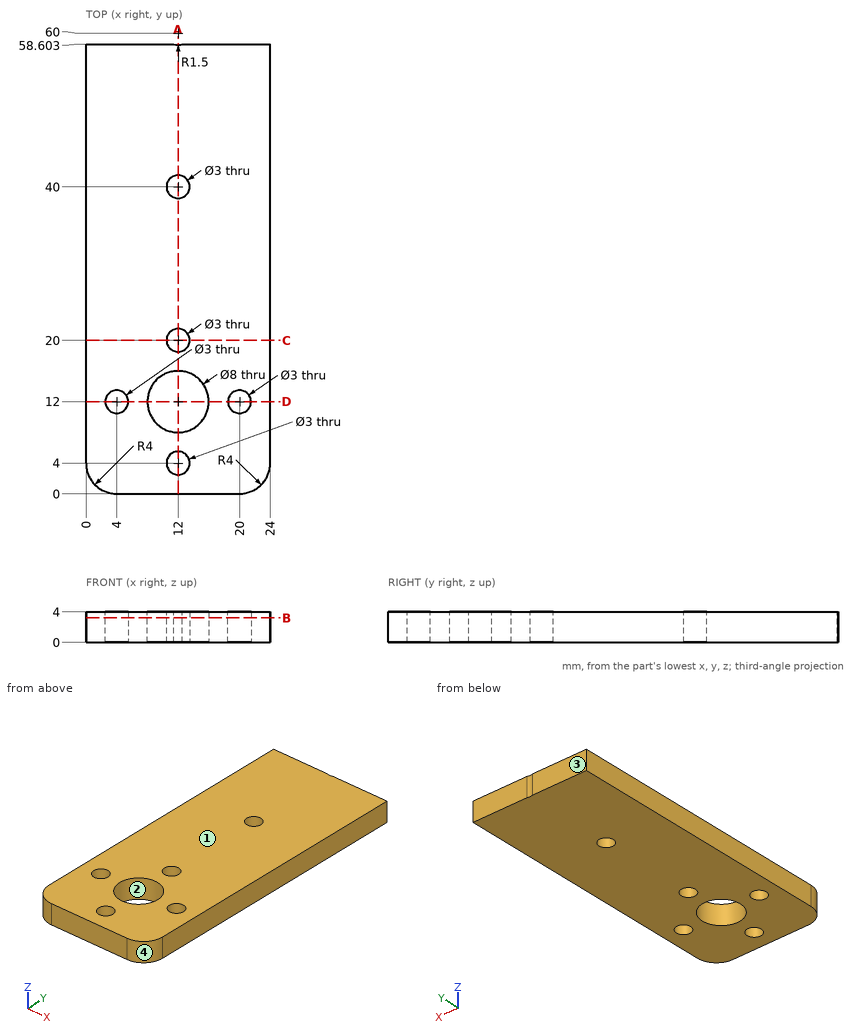
For this review, use the dimensioned drawing (mm, ordinates from the lowest corner) and the shaded views. Round coordinates to 2 decimals unless told otherwise and drop trailing zeros. Order: outer loops, then holes, each group sorted by start corner. A loop starts at its lowest first (then second) coordinate and runs counter-clockwise, first axis right, second up.
1) For L1, parallel to Y at x = 12, z = 2.4; L2, parallel to Y at x = 20, z = 1.65; L3, parallel to X at y = 11, z = 3.4, list the stretches that pass through material, from the lowest coordinate up.
The answers:
L1: y = 0 to 2.5, 5.5 to 8, 16 to 18.5, 21.5 to 38.5, 41.5 to 58.5
L2: y = 0 to 10.5, 13.5 to 58.6
L3: x = 0 to 2.88, 5.12 to 8.13, 15.87 to 18.88, 21.12 to 24
2) Clearance check with a flat-ended pin moving along its axis: pin 1 Ø5 at (x, y) = (12, 40) entering from +Z. State where the tip first meets the part, or that it passes through.
The answers:
pin 1: stops at z = 4
3) Consider section D-D (y = 12). State the section outline as (x, z) points.
The answers:
outline: (0, 0) - (2.5, 0) - (2.5, 4) - (0, 4) - close; (5.5, 0) - (8, 0) - (8, 4) - (5.5, 4) - close; (16, 0) - (18.5, 0) - (18.5, 4) - (16, 4) - close; (21.5, 0) - (24, 0) - (24, 4) - (21.5, 4) - close
4) Consider section A-A (x = 12). State the section outline as (y, z) points.
The answers:
outline: (0, 0) - (2.5, 0) - (2.5, 4) - (0, 4) - close; (5.5, 0) - (8, 0) - (8, 4) - (5.5, 4) - close; (16, 0) - (18.5, 0) - (18.5, 4) - (16, 4) - close; (21.5, 0) - (38.5, 0) - (38.5, 4) - (21.5, 4) - close; (41.5, 0) - (58.5, 0) - (58.5, 4) - (41.5, 4) - close
5) Consider section B-B (z = 3.2). State the section outline as (x, y) points, plus the area to 3 significant figures.
The answers:
outline: (0, 4) arc R4 ccw to (4, 0) - (20, 0) arc R4 ccw to (24, 4) - (24, 58.6) - (12.55, 58.6) arc R1.5 cw to (11.45, 58.6) - (0, 58.6) - close; hole circle Ø3 at (4, 12); hole circle Ø8 at (12, 12); hole circle Ø3 at (12, 4); hole circle Ø3 at (12, 20); hole circle Ø3 at (12, 40); hole circle Ø3 at (20, 12)
area: 1,310 mm2
6) Consider section C-C (y = 20). State the section outline as (x, z) points, plus the area to 3 significant figures.
The answers:
outline: (0, 0) - (10.5, 0) - (10.5, 4) - (0, 4) - close; (13.5, 0) - (24, 0) - (24, 4) - (13.5, 4) - close
area: 84.0 mm2
7) Draft analysis for pull direction Y (two halves, no side actions). For the marked faces 1, 2, 3 and 4, state which applies: released by +Y, released by -Y, zero draft, split by the parting line, or undercut.
The answers:
face 1: zero draft
face 2: undercut
face 3: released by +Y
face 4: released by -Y
